```python
from build123d import *

# Parameters (mm, degrees)
BOSS_EXTRUDE1_DEPTH = 96.52
SKETCH2_W           = 83.82
SKETCH2_H           = 76.2
CUT_EXTRUDE1_DEPTH  = 305.8


with BuildPart() as part:
    # Sketch1 → Boss-Extrude1 (new body)
    with BuildSketch(Plane(origin=(0, 0, 0), x_dir=(0, 0, -1), z_dir=(1, 0, 0))):
        Polygon((0, 0), (12.7, 298.45), (-88.9, 298.45), (-88.9, 304.8), (101.6, 304.8), (101.6, 0), align=None)
    extrude(amount=BOSS_EXTRUDE1_DEPTH)

    # Sketch2 → Cut-Extrude1 (cut, through all)
    with BuildSketch(Plane.XZ):
        with Locations((48.26, -57.15)):
            Rectangle(SKETCH2_W, SKETCH2_H)
    extrude(amount=-CUT_EXTRUDE1_DEPTH, mode=Mode.SUBTRACT)


solid = part.part
```
Model file for the job. Use its own axes, mm. A direction names the side the tool comes from. Coordinates: 2 decimals unless noted, no trailing zeros. Write each loop counter-clockwise with the first axis right and the second up, starting at its lowest first coordinate (ties: lowest second). Pieces come first, ordered by that corner, then holes. Notation, with made-up numbers: (75, -10) - (79, -10) arc R22 cw to (79, 26) - close; hole circle Ø2 at (10, 73). An arc over 180 degrees is marked (long way). One line per item, written item: value. Start each with the question number.
1. Mould opens along Y. For faces 1 (the flat face through (48, 304.8, 16)), 2 (the flat face through (48, 150, -19.05)), 3 (the flat face through (47.58, 147.14, -6.26)) say: released by +Y, released by -Y, zero draft, split by the parting line, or undercut.
2. Tool access for faces 4 (the flat face through (48, 302, 88.9)), 5 (the flat face through (48, 150, -95.25)): list every direction of +Z, -Z, +X, -X, +Y, -Y with a clear straight run to the whole face (end or side of a thin tool).
3. Slice it at D-D (y = 247). Write the cut outline in (x, z).
4. Slice it at A-A (z = -74.5). Write the cut outline in (x, y).
5. Flat gauge pins, fed straight in: pin 1 (6 mm diameter, centred on x = 42, y = 148.5, fed in from +Z); pin 2 (5 mm diameter, centred on x = 42, y = 161, fed in from +Z); pin 3 (25 mm diameter, centred on x = 41, y = 124.5, fed in from +Z); pin 4 (2 mm diameter, centred on y = 116, z = -8.5, fed in from -X). Where does each tip first touch, or does it go through?
6. Probe line 1 (X direction, y = 103.5, z = -55); line 2 (Y direction, x = 85, z = 22.5); line 3 (Z direction, x = 20.5, y = 42.5). List the from-to ranges inside material, lowest first. Write a range as from..to.
7. Slice it at B-B (x = 16). Write the cut outline in (y, z).
8. Slice it at C-C (y = 40.5). Write the cut outline in (x, z), plus the area to 3 significant figures.
Answers below:
1. face 1: released by +Y
1. face 2: zero draft
1. face 3: undercut
2. face 4: +Z, +X, -X, +Y, -Y
2. face 5: +Y, -Y
3. outline: (0, -101.6) - (96.52, -101.6) - (96.52, -10.51) - (0, -10.51) - close; hole (6.35, -95.25) - (90.17, -95.25) - (90.17, -19.05) - (6.35, -19.05) - close
4. outline: (0, 0) - (6.35, 0) - (6.35, 304.8) - (0, 304.8) - close; (90.17, 0) - (96.52, 0) - (96.52, 304.8) - (90.17, 304.8) - close
5. pin 1: stops at z = -6.19
5. pin 2: stops at z = -6.74
5. pin 3: stops at z = -4.77
5. pin 4: stops at x = 0
6. line 1: x = 0..6.35, 90.17..96.52
6. line 2: y = 298.45..304.8
6. line 3: z = -101.6..-95.25, -19.05..-1.81
7. outline: (0, -101.6) - (304.8, -101.6) - (304.8, -95.25) - (0, -95.25) - close; (0, -19.05) - (304.8, -19.05) - (304.8, 88.9) - (298.45, 88.9) - (298.45, -12.7) - (0, 0) - close
8. outline: (0, -101.6) - (96.52, -101.6) - (96.52, -1.72) - (0, -1.72) - close; hole (6.35, -95.25) - (90.17, -95.25) - (90.17, -19.05) - (6.35, -19.05) - close
8. area: 3,250 mm^2
